Input: part model. Units: mm. Frame: model coordinates. A direction names the side the tool comes from. Give positions to 0.01 mm unless a question says otherwise; leave off trailing zeros. Write each loop counter-clockwise with the first axis right and the second up, starting at its lowest first coordinate (ties: lowest second). Pieces come first, ordered by that corner, then holes.
```python
from build123d import *

# Parameters (mm, degrees)
SKICA1_R        = 3
SKICA1_R_2      = 1.5
VYSUNOUT1_DEPTH = 4
VYSUNOUT2_START = -1.5
SKICA2_R        = 4.5
SKICA2_R_2      = 3
VYSUNOUT2_DEPTH = 1.5
ZAOBLIT1_R      = 0.45
ZKOSIT1_SIZE    = 0.3


with BuildPart() as part:
    # Skica1 → Vysunout1 (new body)
    with BuildSketch(Plane.XY):
        Circle(SKICA1_R)
        Circle(SKICA1_R_2, mode=Mode.SUBTRACT)
    extrude(amount=VYSUNOUT1_DEPTH)

    # Skica2 → Vysunout2 (add)
    with BuildSketch(Plane.XY.offset(4).offset(VYSUNOUT2_START)):
        Circle(SKICA2_R)
        Circle(SKICA2_R_2, mode=Mode.SUBTRACT)
    extrude(amount=VYSUNOUT2_DEPTH)

    # Zaoblit1
    zaoblit1_edges = [part.edges().sort_by_distance(p)[0] for p in [
        (-3, 0, 2.5),
    ]]
    fillet(zaoblit1_edges, radius=ZAOBLIT1_R)

    # Zkosit1
    zkosit1_edges = [part.edges().sort_by_distance(p)[0] for p in [
        (-4.5, 0, 2.5),
        (-4.5, 0, 4),
        (-3, 0, 0),
        (-1.5, 0, 0),
        (-1.5, 0, 4),
    ]]
    chamfer(zkosit1_edges, length=ZKOSIT1_SIZE)


solid = part.part
```
Q1. Section C-C, the plane z = 1.15. Return the cut outline in (x, y), then the cut area to 3 significant figures.
Q2. Pin query (flat end, axial travel): pin 1 (2.5 mm diameter, centred on x = 0, y = 0, fed in from +Z); pin 2 (1.5 mm diameter, centred on y = -2.5, z = 2, fed in from +X); pin 3 (1 mm diameter, centred on x = -2.5, z = 1, fed in from -Y); pin 4 (5 mm diameter, centred on x = -1, y = -1, fed in from -Z). Return the tip coordinate at first contact, or that it passes through.
Q3. Section A-A, the plane y = 0. Return the cut outline in (x, z), then the cut area to 3 significant figures.
Q4. Material intervals for line 1 along Z through (x, y) = (-3.5, -2); line 2 along Y through (x, z) = (0, 2.4); line 3 along Y through (x, z) = (0, 2.3), sorted ascending.
Q5. Mould query, pull axis Y, two halves, no side actions, for faces 3 (the cylindrical face through (-3, 0, 1)), 4 (the flat face through (2, -1, 0)), 5 (the cylindrical face through (-1.5, 0.07, 1.98)). Classes: +Y half, -Y half, draft (parallel to the pull), parting line (faces both ways), or undercut.
Q6. Access query for faces 1 (the flat face through (-3, 2, 2.5)), 2 (the flat face through (2, 0, 4)). Directions: +Z, -Z, +X, -X, +Y, -Y. A direction counts if a zero-diameter tool reaches every point of the face in a straight line with its end or side. Return the directions, or none.
Solutions:
1. outline: circle Ø6 at (0, 0); hole circle Ø3 at (0, 0)
1. area: 21.2 mm2
2. pin 1: passes through
2. pin 2: stops at x = 3.8
2. pin 3: stops at y = -2.24
2. pin 4: stops at z = 0
3. outline: (-4.5, 2.8) - (-4.2, 2.5) - (-3.45, 2.5) arc R0.45 cw to (-3, 2.05) - (-3, 0.3) - (-2.7, 0) - (-1.8, 0) - (-1.5, 0.3) - (-1.5, 3.7) - (-1.8, 4) - (-4.2, 4) - (-4.5, 3.7) - close; (1.5, 0.3) - (1.8, 0) - (2.7, 0) - (3, 0.3) - (3, 2.05) arc R0.45 cw to (3.45, 2.5) - (4.2, 2.5) - (4.5, 2.8) - (4.5, 3.7) - (4.2, 4) - (1.8, 4) - (1.5, 3.7) - close
3. area: 16.1 mm2
4. line 1: z = 2.5 to 4
4. line 2: y = -3.17 to -1.5, 1.5 to 3.17
4. line 3: y = -3.08 to -1.5, 1.5 to 3.08
5. face 3: parting line
5. face 4: draft
5. face 5: undercut
6. face 1: -Z
6. face 2: +Z, +X, -X, +Y, -Y
